```python
from build123d import *

# Parameters (mm, degrees)
SKETCH1_W           = 110
SKETCH1_H           = 76
BOSS_EXTRUDE1_DEPTH = 35
SKETCH2_W           = 15
SKETCH2_H           = 74
SKETCH2_W_2         = 5
CUT_EXTRUDE1_DEPTH  = 32
SKETCH3_W           = 11.235183257
SKETCH3_H           = 58.560748925
BOSS_EXTRUDE2_DEPTH = 17
SKETCH4_W           = 85.227436201
SKETCH4_H           = 71.879332631
BOSS_EXTRUDE3_DEPTH = 1
SKETCH5_W           = 90
SKETCH5_H           = 76
BOSS_EXTRUDE4_DEPTH = 22
SKETCH6_R           = 7.5
BOSS_EXTRUDE5_DEPTH = 15
SKETCH7_R           = 1.6
CUT_EXTRUDE2_DEPTH  = 5


with BuildPart() as part:
    # Sketch1 → Boss-Extrude1 (new body)
    with BuildSketch(Plane.XY):
        Rectangle(SKETCH1_W, SKETCH1_H)
    extrude(amount=BOSS_EXTRUDE1_DEPTH)

    # Sketch2 → Cut-Extrude1 (cut)
    with BuildSketch(Plane.XY.offset(35)):
        with Locations((47.5, -1)):
            Rectangle(SKETCH2_W, SKETCH2_H)
        with Locations((-52.5, -1)):
            Rectangle(SKETCH2_W_2, SKETCH2_H)
    extrude(amount=-CUT_EXTRUDE1_DEPTH, mode=Mode.SUBTRACT)

    # Sketch3 → Boss-Extrude2 (add)
    with BuildSketch(Plane.XY.offset(3)):
        with Locations((45.617591629, 0.154641352)):
            Rectangle(SKETCH3_W, SKETCH3_H)
    extrude(amount=BOSS_EXTRUDE2_DEPTH)

    # Sketch4 → Boss-Extrude3 (add)
    with BuildSketch(Plane.XY.offset(35)):
        with Locations((-4.69027722, 0.263838975)):
            Rectangle(SKETCH4_W, SKETCH4_H)
    extrude(amount=BOSS_EXTRUDE3_DEPTH)

    # Sketch5 → Boss-Extrude4 (add)
    with BuildSketch(Plane.XY.offset(36)):
        with Locations((-5, 0)):
            Rectangle(SKETCH5_W, SKETCH5_H)
    extrude(amount=BOSS_EXTRUDE4_DEPTH)

    # Sketch6 → Boss-Extrude5 (add)
    with BuildSketch(Plane.XZ.offset(38)):
        with Locations(Location((-5, 48.2, 0), (0, 0, 270))):
            Circle(SKETCH6_R)
        with Locations(Location((11, 48.2, 0), (0, 0, 90))):
            Circle(SKETCH6_R)
        with Locations(Location((27, 48.2, 0), (0, 0, 90))):
            Circle(SKETCH6_R)
        with Locations(Location((-21, 48.2, 0), (0, 0, 90))):
            Circle(SKETCH6_R)
        with Locations(Location((-37, 48.2, 0), (0, 0, 90))):
            Circle(SKETCH6_R)
    extrude(amount=BOSS_EXTRUDE5_DEPTH)

    # Sketch7 → Cut-Extrude2 (cut)
    with BuildSketch(Plane.XZ.offset(-36)):
        with Locations(Location((50, 27.5, 0), (0, 0, 270))):
            Circle(SKETCH7_R)
        with BuildLine():
            Line((-55, 29.1), (-52.6, 29.1))
            ThreePointArc((-52.6, 29.1), (-51, 27.5), (-52.6, 25.9))
            Line((-52.6, 25.9), (-55, 25.9))
            Line((-55, 25.9), (-55, 29.1))
        make_face()
    extrude(amount=-CUT_EXTRUDE2_DEPTH, mode=Mode.SUBTRACT)


solid = part.part
```
Could you check a few things on this model? Use its own coordinates, in mm. A direction names the side the tool comes from. Round coordinates to 2 decimals unless told otherwise and drop trailing zeros. Loops run counter-clockwise (first coordinate to the right, second up) from the corner with the lowest first, then second, coordinate; pieces in that order, holes last. Notation, with made-up numbers: (20.25, -26) - (64.25, -26) arc R36 cw to (64.25, 9) - close; hole circle Ø9 at (-36, 73). An arc over 180 degrees is marked (long way). Answer in a Markdown table with one row per item. Add a question column.
(1) If we section it at B-B (z = 27.5): Please give me the cut outline in (x, y).
(2) I need wall thicknesses on line 1 along X through (y, z) = (37.45, 27.5); line 2 along Y through (x, z) = (46, 10); line 3 along X through (y, z) = (-25.5, 36.5). Which ranges of each line are inside material? Lowest first, please.
(3) If we section it at C-C (x = 27): Please give me the cut outline in (y, z), plus the area to 3 significant figures.
(4) If we mould it in two halves opening along Y, with no side actions, what happens to faces 1 (the face through (52, 0, 3)), 2 (the face through (-55, 8, 1)), 3 (the face through (-1, -38, 17))? For each: pulls with the +Y half, pulls with the -Y half, needs draft (parallel to the pull), parting line crosses it, or undercut.
(5) If we section it at D-D (y = -4): Please give me the cut outline in (x, z).
(6) If we section it at A-A (x = 50): Please give me the cut outline in (y, z).
(7) For faces 4 (the face through (-9, -36, 36)), 5 (the face through (-50, -2, 19)), 6 (the face through (-2.747, -45.395, 41.046)), 7 (the face through (40, -1, 47)), which set-ups out of +Z, -Z, +X, -X, +Y, -Y let a thin tool reach every point of the face, with its end or its side?
(8) I'm going to push flat-ended pins straight in: pin 1 (0.5 mm diameter, centred on y = 4, z = 35.5, fed in from -X); pin 2 (10 mm diameter, centred on y = -15.5, z = 17.5, fed in from -X); pin 3 (9 mm diameter, centred on x = 47.5, y = 10, fed in from +Z). Where does each tip first touch, or does it pass through?
Model answer:
| question | item | result |
|---|---|---|
| 1 | outline | (-51, 36) - (-50, 36) - (-50, -38) - (40, -38) - (40, 36) - (48.4, 36) - (48.4, 38) - (-51, 38) - close; (51.6, 36) - (55, 36) - (55, 38) - (51.6, 38) - close |
| 2 | line 1 | x = -51 to 48.4, 51.6 to 55 |
| 2 | line 2 | y = -29.13 to 29.44, 36 to 38 |
| 2 | line 3 | x = -50 to 40 |
| 3 | outline | (-53, 40.7) - (-38, 40.7) - (-38, 36) - (-35.68, 36) - (-35.68, 35) - (-38, 35) - (-38, 0) - (38, 0) - (38, 35) - (36.2, 35) - (36.2, 36) - (38, 36) - (38, 58) - (-38, 58) - (-38, 55.7) - (-53, 55.7) - close |
| 3 | area | 4,630 mm² |
| 4 | face 1 | undercut |
| 4 | face 2 | needs draft |
| 4 | face 3 | pulls with the -Y half |
| 5 | outline | (-55, 0) - (55, 0) - (55, 3) - (51.24, 3) - (51.24, 20) - (40, 20) - (40, 35) - (37.92, 35) - (37.92, 36) - (40, 36) - (40, 58) - (-50, 58) - (-50, 36) - (-47.3, 36) - (-47.3, 35) - (-50, 35) - (-50, 3) - (-55, 3) - close |
| 6 | outline | (-38, 0) - (38, 0) - (38, 25.9) - (36, 25.9) - (36, 3) - (29.44, 3) - (29.44, 20) - (-29.13, 20) - (-29.13, 3) - (-38, 3) - close; (36, 29.1) - (38, 29.1) - (38, 35) - (36, 35) - close |
| 7 | face 4 | none |
| 7 | face 5 | +Z, -X, -Y |
| 7 | face 6 | -Y |
| 7 | face 7 | +Z, +X, +Y, -Y |
| 8 | pin 1 | stops at x = -47.3 |
| 8 | pin 2 | stops at x = -50 |
| 8 | pin 3 | stops at z = 20 |
